Input: part model. Units: mm. Frame: model coordinates. A direction names the side the tool comes from. Round coordinates to 2 decimals unless told otherwise and drop trailing zeros. Answer as a JSON object with one key per item and string values.
```python
from build123d import *

# Parameters (mm, degrees)
ESQUISSE1_W             = 480
ESQUISSE1_H             = 296
BOSS_EXTRU_1_DEPTH      = 13
ESQUISSE2_W             = 130
ESQUISSE2_H             = 130
ESQUISSE3_W             = 460
ESQUISSE3_H             = 276
ENL_V_MAT_EXTRU_1_DEPTH = 2
CONG_1_R                = 15
ESQUISSE4_W             = 200
ESQUISSE4_H             = 53.029675638
ENL_V_MAT_EXTRU_2_DEPTH = 61.0000001
ESQUISSE5_W             = 15
ESQUISSE5_H             = 5
BOSS_EXTRU_2_DEPTH      = 1


with BuildPart() as part:
    # Esquisse1 → Boss.-Extru.1 (new body)
    with BuildSketch(Plane.XY):
        Rectangle(ESQUISSE1_W, ESQUISSE1_H)
    extrude(amount=BOSS_EXTRU_1_DEPTH)

    # Esquisse2 → section 0 of lissage1
    with BuildSketch(Plane.XY.offset(45), mode=Mode.PRIVATE) as lissage1_s0:
        Rectangle(ESQUISSE2_W, ESQUISSE2_H)
    # loft up to a face of the part (lissage1)
    loft([lissage1_s0.sketch, part.faces().sort_by_distance((0, 0, 13))[0]])

    # Esquisse3 → Enlèv. mat.-Extru.1 (cut)
    with BuildSketch(Plane(origin=(0, 0, 0), x_dir=(-1, 0, 0), z_dir=(0, 0, -1))):
        Rectangle(ESQUISSE3_W, ESQUISSE3_H)
    extrude(amount=-ENL_V_MAT_EXTRU_1_DEPTH, mode=Mode.SUBTRACT)

    # Congé1
    cong_1_edges = [part.edges().sort_by_distance(p)[0] for p in [
        (-240, 148, 6.5),
        (240, 148, 6.5),
        (240, -148, 6.5),
        (-240, -148, 6.5),
    ]]
    fillet(cong_1_edges, radius=CONG_1_R)

    # Esquisse4 → Enlèv. mat.-Extru.2 (cut, through all)
    with BuildSketch(Plane(origin=(0, 88, 0), x_dir=(1, 0, 0), z_dir=(0, 1, 0))):
        with Locations((0, -41.514837819)):
            Rectangle(ESQUISSE4_W, ESQUISSE4_H)
    extrude(amount=ENL_V_MAT_EXTRU_2_DEPTH, mode=Mode.SUBTRACT)

    # Esquisse5 → Boss.-Extru.2 (add)
    with BuildSketch(Plane(origin=(0, 0, 0), x_dir=(-1, 0, 0), z_dir=(0, 0, -1))):
        with Locations((-208.124292846, 143.5)):
            Rectangle(ESQUISSE5_W, ESQUISSE5_H)
        with Locations((-185.124292846, 143.5)):
            Rectangle(ESQUISSE5_W, ESQUISSE5_H)
        with Locations((-162.124292846, 143.5)):
            Rectangle(ESQUISSE5_W, ESQUISSE5_H)
    extrude(amount=BOSS_EXTRU_2_DEPTH)


solid = part.part
```
1) Ray query, probe 1 along Z at (x, y) = (0.5, 132); probe 2 along Z at (x, y) = (61.5, -29.5). Return the intervals inside material, ascending.
Output:
{"probe 1": "z = 2 to 15", "probe 2": "z = 2 to 45"}
2) Contact query for flat-ended pins moving along their axis: P1, Ø8, axis at x = 142, y = 5.5, coming from the -Z side; P2, Ø0.8, axis at x = 204.5, z = -0.5, coming from the +Y side; P3, Ø6.5, axis at y = 124, z = 27, coming from the +X side. Output: stop coordinate, or through.
Output:
{"P1": "stops at z = 2", "P2": "stops at y = 146", "P3": "passes through"}
3) Reachability of faces 1 (the face through (-240, -2, 6)), 2 (the face through (100, 103, 21)) from +Z, -Z, +X, -X, +Y, -Y: full face, straight path, thin tool, end or side. Return the list, or none.
Output:
{"face 1": "+Z, -Z, -X, +Y, -Y", "face 2": "+Z, +Y"}
4) Draft query along Y for faces 3 (the face through (3, 2, 2)), 4 (the face through (-235.72, 143.49, 7.16)), 5 (the face through (-3, -148, 6)), 6 (the face through (-1, 115, 15)). Return one class per face: +Y half, -Y half, draft (parallel to the pull), parting line (faces both ways), or undercut.
Output:
{"face 3": "undercut", "face 4": "+Y half", "face 5": "-Y half", "face 6": "draft"}
